Design review of the part built by this model. Coordinates are the model's own, in mm. A direction names the side the tool comes from. Give positions to 0.01 mm unless a question says otherwise; leave off trailing zeros. Write each loop counter-clockwise with the first axis right and the second up, starting at its lowest first coordinate (ties: lowest second). Pieces come first, ordered by that corner, then holes. Notation, with made-up numbers: (56, 4.25) - (72, 4.25) arc R16 cw to (72, 18.25) - close; hole circle Ø7 at (35, -33.75). An arc over 180 degrees is marked (long way). Write each question's results on one line, items separated by ' | '. Start each with the question number.
from build123d import *

# Parameters (mm, degrees)
SKETCH1_W                   = 21.59
SKETCH1_H                   = 13.208
BOSS_EXTRUDE1_DEPTH         = 1.6
F_44_0_086_DIAMETER_HOLE1_D = 2.1844
SKETCH4_W                   = 7
SKETCH4_H                   = 7.2
BOSS_EXTRUDE2_DEPTH         = 3.1


with BuildPart() as part:
    # Sketch1 → Boss-Extrude1 (new body)
    with BuildSketch(Plane(origin=(0, 0, 0), x_dir=(0, 0, -1), z_dir=(1, 0, 0))):
        with Locations((10.795, 6.604)):
            Rectangle(SKETCH1_W, SKETCH1_H)
    extrude(amount=BOSS_EXTRUDE1_DEPTH)

    # #44 (0.086) Diameter Hole1 (through all)
    with Locations(Plane(origin=(1.6, 0, 0), x_dir=(0, 0, -1), z_dir=(1, 0, 0))):
        with Locations((1.905, 11.049), (19.685, 11.049), (19.685, 2.159), (1.905, 2.159)):
            Hole(F_44_0_086_DIAMETER_HOLE1_D / 2)

    # Sketch4 → Boss-Extrude2 (add)
    with BuildSketch(Plane(origin=(1.6, 0, 0), x_dir=(0, 0, -1), z_dir=(1, 0, 0))):
        with Locations((10.795, 10.108)):
            Rectangle(SKETCH4_W, SKETCH4_H)
    extrude(amount=BOSS_EXTRUDE2_DEPTH)


solid = part.part
Q1. Add section D-D on z = -9. State the section outline as (x, y) points.
Q2. Machinability: for faces 4 (the face through (3, 6.508, -11)), 5 (the face through (0, 7, -11)), 6 (the face through (1, 13.208, -11)), 7 (the face through (3, 10, -14.295)), 8 (the face through (3, 10, -7.295)), which of the approach directions +Z, -Z, +X, -X, +Y, -Y give a long, thin tool a straight path to every point of the face, cutting with its end or side? Answer none if there is none.
Q3. For line 1 along Z through (x, y) = (1.25, 11); line 2 along Y through (x, z) = (0.75, -2.25); line 3 along Z through (x, y) = (2.8, 10.5) (3 decimals), list the stretches that pass through material, from the lowest coordinate up. Write a range as [from, to].
Q4. Add section A-A on y = 8. State the section outline as (x, z) points (3 decimals).
Q5. Add section B-B on z = -20. State the section outline as (x, y) points, plus the area to 3 significant figures.
Q6. Add section C-C on x = 0.7. State the section outline as (y, z) points (3 decimals), plus the area to 3 significant figures.
Q7. The part is to be moulded in two halves that separate along Z. For faces 1 (the face through (4.7, 10, -11)), 2 (the face through (0.79, 1.49, -20.55)), 3 (the face through (1, 7, 0)), say which applies: +Z half, -Z half, draft (parallel to the pull), parting line (faces both ways), or undercut.
Q8. Insertion check: P1, Ø0.9, axis at x = 3, y = 9, coming from the -Z side (3 decimals); P2, Ø0.9, axis at x = 3, y = 10.5, coming from the +Z side (3 decimals); P3, Ø3.5, axis at y = 2.159, z = -19.685, coming from the +X side. Each pin has a flat end and moves straight along its axis. Give the tip position at first contact, or say it passes through.
Result:
1) outline: (0, 0) - (1.6, 0) - (1.6, 6.51) - (4.7, 6.51) - (4.7, 13.71) - (1.6, 13.71) - (1.6, 13.21) - (0, 13.21) - close
2) face 4: +Z, -Z, +X, -Y | face 5: +Z, -Z, -X, +Y, -Y | face 6: +Z, -Z, -X, +Y | face 7: -Z, +X, +Y, -Y | face 8: +Z, +X, +Y, -Y
3) line 1: z = [-21.59, -20.78], [-18.59, -3], [-0.81, 0] | line 2: y = [0, 1.12], [3.2, 10.01], [12.09, 13.21] | line 3: z = [-14.295, -7.295]
4) outline: (0, -21.59) - (1.6, -21.59) - (1.6, -14.295) - (4.7, -14.295) - (4.7, -7.295) - (1.6, -7.295) - (1.6, 0) - (0, 0) - close
5) outline: (0, 0) - (1.6, 0) - (1.6, 1.11) - (0, 1.11) - close; (0, 3.2) - (1.6, 3.2) - (1.6, 10) - (0, 10) - close; (0, 12.09) - (1.6, 12.09) - (1.6, 13.21) - (0, 13.21) - close | area: 14.4 mm²
6) outline: (0, -21.59) - (13.208, -21.59) - (13.208, 0) - (0, 0) - close; hole circle Ø2.184 at (2.159, -19.685); hole circle Ø2.184 at (2.159, -1.905); hole circle Ø2.184 at (11.049, -19.685); hole circle Ø2.184 at (11.049, -1.905) | area: 270 mm²
7) face 1: draft | face 2: undercut | face 3: +Z half
8) P1: stops at z = -14.295 | P2: stops at z = -7.295 | P3: stops at x = 1.6
